Geometry: final body of the model. Coordinates: model frame, mm. Round coordinates to 2 decimals unless told otherwise and drop trailing zeros. Write each loop counter-clockwise with the first axis right and the second up, starting at its lowest first coordinate (ties: lowest second). Pieces come first, ordered by that corner, then holes. Notation, with made-up numbers: (37.25, -19) -> (72.25, -19) arc R8 cw to (72.25, -14) -> close; hole circle Ø2 at (-15.75, -33.75). An arc over 180 degrees is marked (long way). Use one line per item in the form item = value. Start each with the question number.
1. Cut plane D-D, the plane x = 10.5. Return the cut outline in (y, z).
2. Cut plane C-C, the plane z = 0. Return the cut outline in (x, y), plus the area to 3 significant figures.
3. Cut plane B-B, the plane y = 0. Return the cut outline in (x, z), plus the area to 3 significant figures.
4. Line query: L1, parallel to Z at x = 7, y = -0.05; L2, parallel to Z at x = 13.5, y = 0; L3, parallel to X at y = -0.05, z = 0. Output: solid intervals per line, ascending.
5. Cut plane A-A, the plane x = 13.75. Return the cut outline in (y, z), plus the area to 3 significant figures.
```python
from build123d import *

# Parameters (mm, degrees)
SKETCH1_R           = 4
BOSS_EXTRUDE1_DEPTH = 0.1
SKETCH2_W           = 12
SKETCH2_H           = 6
BOSS_EXTRUDE2_DEPTH = 0.1
SKETCH3_W           = 5
SKETCH3_H           = 1
BOSS_EXTRUDE3_DEPTH = 0.1


with BuildPart() as part:
    # Sketch1 → Boss-Extrude1 (new body, symmetric)
    with BuildSketch(Plane(origin=(0, 0, 0), x_dir=(1, 0, 0), z_dir=(0, 1, 0))):
        Circle(SKETCH1_R)
    extrude(amount=BOSS_EXTRUDE1_DEPTH, both=True)

    # Sketch2 → Boss-Extrude2 (add, symmetric)
    with BuildSketch(Plane(origin=(0, 0, 0), x_dir=(1, 0, 0), z_dir=(0, 1, 0))):
        with Locations((6, 0)):
            Rectangle(SKETCH2_W, SKETCH2_H)
    extrude(amount=BOSS_EXTRUDE2_DEPTH, both=True)

    # Sketch3 → Boss-Extrude3 (add, symmetric)
    with BuildSketch(Plane(origin=(0, 0, 0), x_dir=(1, 0, 0), z_dir=(0, 1, 0))):
        with Locations((14.5, 1)):
            Rectangle(SKETCH3_W, SKETCH3_H)
    boss_extrude3 = extrude(amount=BOSS_EXTRUDE3_DEPTH, both=True)

    # Mirror1: Boss-Extrude3 across plane
    add(boss_extrude3.mirror(Plane.XY))


solid = part.part
```
Outcome:
q1.outline = (-0.1, -3) -> (0.1, -3) -> (0.1, 3) -> (-0.1, 3) -> close
q2.outline = (-4, -0.1) -> (12, -0.1) -> (12, 0.1) -> (-4, 0.1) -> close
q2.area = 3.20 mm^2
q3.outline = (2.65, -3) -> (12, -3) -> (12, -1.5) -> (17, -1.5) -> (17, -0.5) -> (12, -0.5) -> (12, 0.5) -> (17, 0.5) -> (17, 1.5) -> (12, 1.5) -> (12, 3) -> (2.65, 3) arc R4 ccw (long way) to start
q3.area = 111 mm^2
q4.L1 = -3 to 3
q4.L2 = -1.5 to -0.5, 0.5 to 1.5
q4.L3 = -4 to 12
q5.outline = (-0.1, -1.5) -> (0.1, -1.5) -> (0.1, -0.5) -> (-0.1, -0.5) -> close; (-0.1, 0.5) -> (0.1, 0.5) -> (0.1, 1.5) -> (-0.1, 1.5) -> close
q5.area = 0.400 mm^2
